Read the model definition and answer for the solid it produces. Units are mm, in the model's axes. A direction names the side the tool comes from. Coordinates: 2 decimals unless noted, no trailing zeros. Loops run counter-clockwise (first coordinate to the right, second up) from the corner with the lowest first, then second, coordinate; pieces in that order, holes last.
from build123d import *

# Parameters (mm, degrees)
BOSS_EXTRUDE3_DEPTH = 38
BOSS_EXTRUDE4_DEPTH = 6


with BuildPart() as part:
    # Sketch1 → Boss-Extrude3 (new body)
    with BuildSketch(Plane.XY):
        Polygon((-107.68463, 30.25), (107.648903001, 30.25), (132.321905897, -15.300159192), (135.572573725, -21.301392104), (142.39764743, -21.30397981), (111.222575033, 36.25), (-111.260793608, 36.25), (-142.331864382, -21.196025493), (-135.511854399, -21.198611279), (-132.267274575, -15.19984102), align=None)
    extrude(amount=BOSS_EXTRUDE3_DEPTH)

    # Sketch1_3 → Boss-Extrude4 (add)
    with BuildSketch(Plane.XY):
        Polygon((-107.68463, 30.25), (107.648903001, 30.25), (132.321905897, -15.300159192), (135.572573725, -21.301392104), (142.39764743, -21.30397981), (111.222575033, 36.25), (-111.260793608, 36.25), (-142.331864382, -21.196025493), (-135.511854399, -21.198611279), (-132.267274575, -15.19984102), align=None)
        Polygon((135.572573725, -21.301392104), (132.321905897, -15.300159192), (-132.267274575, -15.19984102), (-135.511854399, -21.198611279), align=None)
        Polygon((132.321905897, -15.300159192), (107.648903001, 30.25), (-107.68463, 30.25), (-132.267274575, -15.19984102), align=None)
    boss_extrude4 = extrude(amount=-BOSS_EXTRUDE4_DEPTH)

    # Mirror1: Boss-Extrude4 across plane
    add(boss_extrude4.mirror(Plane(origin=(0, 0, 16), x_dir=(1, 0, 0), z_dir=(0, 0, -1))))


solid = part.part
Q1. Determine the mould class of faces 1 (the face through (-2, 8, 38)), 2 (the face through (127.03, 7.07, 16.31)), 3 (the face through (-2, 5, 32)) for opening direction Z: +Z half, -Z half, draft (parallel to the pull), parting line (faces both ways), or undercut.
Findings below:
face 1: +Z half
face 2: draft
face 3: undercut
Q2. A cutting plane is placed at A-A (y = -8.5). Give the vertices of the cut face in (x, z), then the cut area to 3 significant figures.
Findings below:
outline: (-135.46, -6) - (135.46, -6) - (135.46, 38) - (-135.46, 38) - close; hole (-128.64, 0) - (128.64, 0) - (128.64, 32) - (-128.64, 32) - close
area: 3,690 mm2
Q3. A cutting plane is placed at B-B (x = -18.5). Give the vertices of the cut face in (y, z).
Findings below:
outline: (-21.24, -6) - (36.25, -6) - (36.25, 38) - (-21.24, 38) - (-21.24, 32) - (30.25, 32) - (30.25, 0) - (-21.24, 0) - close
Q4. Flat-ended cylindrical pins translate along their axes: pin 1 Ø4 at (y, z) = (-12, 25) entering from +X; pin 2 Ø10 at (y, z) = (24, 6.5) entering from -X; pin 3 Ø8 at (y, z) = (30.5, 14) entering from -X. Find the tip coordinate at first contact, or state that the pin passes through.
Findings below:
pin 1: stops at x = 138.44
pin 2: stops at x = -120.59
pin 3: stops at x = -116.53
Q5. Which of the six approach directions +Z, -Z, +X, -X, +Y, -Y give full straight-line access (tool end or side, diameter ignored) to faces 4 (the face through (-2, 30.25, 16)), 5 (the face through (-126.58, 7.93, 16.31))?
Findings below:
face 4: -Y
face 5: +Z, -Z, -X, +Y
Q6. A cutting plane is placed at C-C (z = 26.5). Give the vertices of the cut face in (x, y).
Findings below:
outline: (-142.33, -21.2) - (-135.51, -21.2) - (-107.68, 30.25) - (107.65, 30.25) - (135.57, -21.3) - (142.4, -21.3) - (111.22, 36.25) - (-111.26, 36.25) - close
Q7. A cutting plane is placed at D-D (y = 6). Give the vertices of the cut face in (x, z), then the cut area to 3 significant figures.
Findings below:
outline: (-127.62, -6) - (127.61, -6) - (127.61, 38) - (-127.62, 38) - close; hole (-120.8, 0) - (120.78, 0) - (120.78, 32) - (-120.8, 32) - close
area: 3,500 mm2
Q8. Straight lines are drawn through the part: probe 1 along Z at (x, y) = (101.5, -17.5); probe 2 along Y at (x, z) = (-77, 22); probe 3 along X at (y, z) = (10, 20). For each, find the intervals that lie inside material, in ascending order.
Findings below:
probe 1: z = -6 to 0, 32 to 38
probe 2: y = 30.25 to 36.25
probe 3: x = -125.46 to -118.64, 118.62 to 125.44
